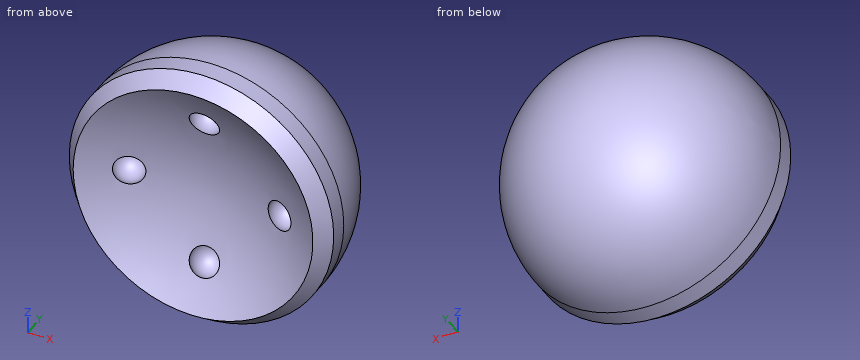
from build123d import *

# Parameters (mm, degrees)
CIRPATTERN2_COUNT = 4


with BuildPart() as part:
    # Sketch1 → Revolve1 (revolve)
    with BuildSketch(Plane.XY):
        with BuildLine():
            Line((-150, 0), (-150, -21.839688718))
            Line((-150, -21.839688718), (-135.992561225, -40.2238734))
            ThreePointArc((-135.992561225, -40.2238734), (-70.908280017, -10.266781974), (0, 0))
            Line((0, 0), (0, 150))
            ThreePointArc((0, 150), (-106.066017178, 106.066017178), (-150, 0))
        make_face()
    revolve(axis=Axis((0, 0, 0), (0, 1, 0)))

    # Sketch2 → Cut-Revolve2 (revolve, cut)
    with BuildSketch(Plane.XY):
        with BuildLine():
            Line((88.925237265, -25.679918596), (88.925237265, 14.320081404))
            ThreePointArc((88.925237265, 14.320081404), (108.925237265, -5.679918596), (88.925237265, -25.679918596))
        make_face()
    cut_revolve2 = revolve(axis=Axis((88.925237265, -25.679918596, 0), (0, 1, 0)), mode=Mode.SUBTRACT)

    # CirPattern2: Cut-Revolve2 ×4 about axis
    cirpattern2_axis = Axis((0, 0, 0), (0, 1, 0))
    for i in range(1, CIRPATTERN2_COUNT):
        add(cut_revolve2.rotate(cirpattern2_axis, i * 360 / CIRPATTERN2_COUNT), mode=Mode.SUBTRACT)


solid = part.part
Model file for the job. Use its own axes, mm. Coordinates: 2 decimals unless noted, no trailing zeros. Write each loop counter-clockwise with the first axis right and the second up, starting at its lowest first coordinate (ties: lowest second). Pieces come first, ordered by that corner, then holes. Notation, with made-up numbers: (83, 59) -> (133, 59) arc R16 ccw to (133, 74) -> close; hole circle Ø10 at (-33, 32.25). An arc over 180 degrees is marked (long way). One line per item, written item: value. Start each with the question number.
1) Slice it at A-A on z = 0. Write the cut outline in (x, y).
2) Probe probe 1 along X at (y, z) = (7, -6); probe 2 along X at (y, z) = (0, -14); probe 3 along X at (y, z) = (-9.5, 95.5). List the from-to ranges inside material, lowest first.
3) Slice it at B-B on x = 0. Write the cut outline in (y, z), then the cut area to 3 significant figures.
4) Flat gauge pins, fed straight in: pin 1 Ø10 at (x, z) = (99.5, 52.5) entering from -Y; pin 2 Ø1.5 at (y, z) = (18.5, 102) entering from -X; pin 3 Ø10 at (x, y) = (46, 68.5) entering from +Z. Where does each tip first touch, or does it go through?
5) Slice it at D-D on y = 98.5. Write the cut outline in (x, z).
6) Slice it at C-C on y = -29. Write the cut outline in (x, z), then the cut area to 3 significant figures.
Answers follow:
1. outline: (-150, -21.84) -> (-135.99, -40.22) arc R250 cw to (-101.26, -21.42) arc R20 cw (long way) to (-69.36, -9.81) arc R250 cw to (69.36, -9.81) arc R20 cw (long way) to (101.26, -21.42) arc R250 cw to (135.99, -40.22) -> (150, -21.84) -> (150, 0) arc R150 ccw to (-150, 0) -> close
2. probe 1: -149.72 to -103.18, -74.67 to 74.67, 103.18 to 149.72
2. probe 2: -149.35 to -102.03, -75.82 to 75.82, 102.03 to 149.35
2. probe 3: -115.67 to -18.5, 18.5 to 115.67
3. outline: (-40.22, -135.99) -> (-21.84, -150) -> (0, -150) arc R150 ccw to (0, 150) -> (-21.84, 150) -> (-40.22, 135.99) arc R250 cw to (-21.42, 101.26) arc R20 cw (long way) to (-9.81, 69.36) arc R250 cw to (-9.81, -69.36) arc R20 cw (long way) to (-21.42, -101.26) arc R250 cw to start
3. area: 37,700 mm2
4. pin 1: y = -29.33
4. pin 2: x = -109.13
4. pin 3: z = 128.42
5. outline: circle Ø226.25 at (0, 0)
6. outline: circle Ø289.09 at (0, 0); hole circle Ø233.74 at (0, 0)
6. area: 22,700 mm2
